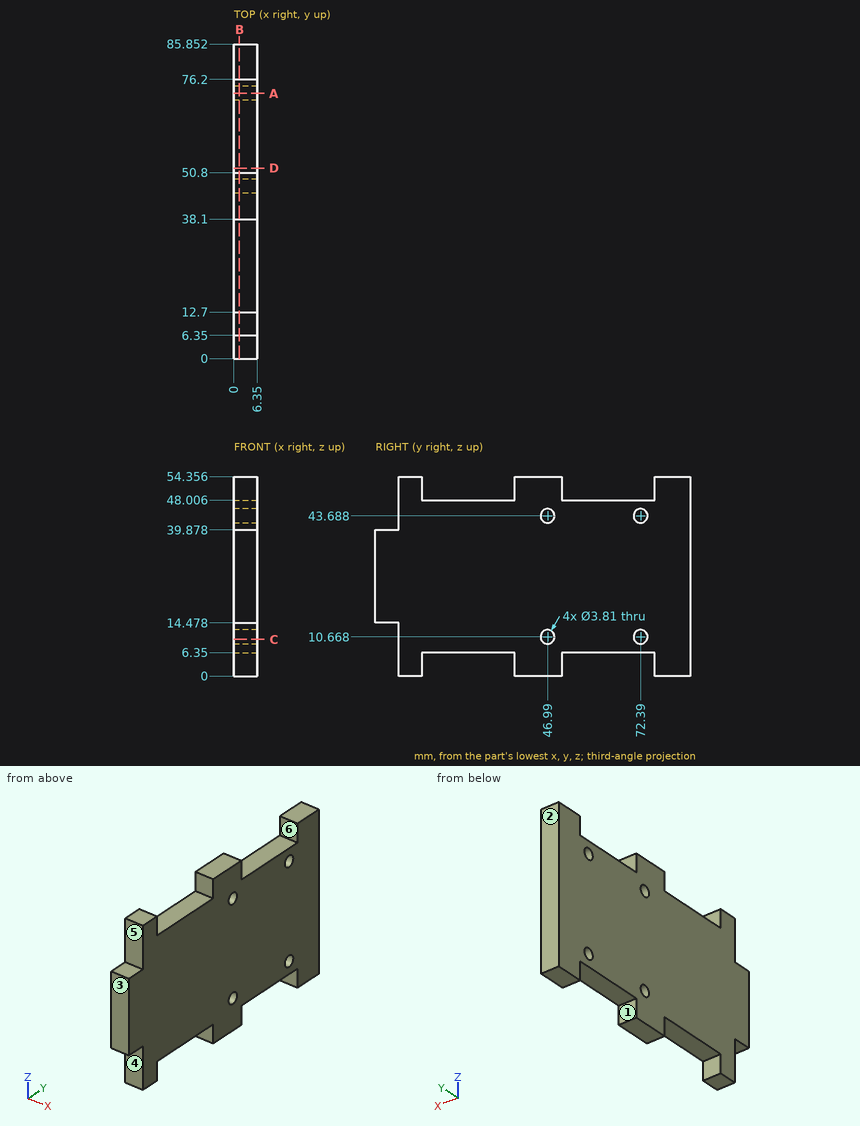
Answer from the drawing. Dimensions are ordinates in mm from the lowest x, y and z of the part. A direction names the side the tool comes from. Round coordinates to 2 decimals unless told otherwise and drop trailing zeros. Write each loop counter-clockwise with the first axis right and the second up, starting at its lowest first coordinate (ties: lowest second). Pieces come first, ordered by that corner, then holes. Notation, with made-up numbers: (32, -12.5) - (78, -12.5) arc R22 ccw to (78, 23.5) - close; hole circle Ø3 at (-12, 74.25). An arc over 180 degrees is marked (long way). Use a Markdown table: item, result.
(1) The part is cut by section A-A (y = 72.39). Write down the section's boundary in (x, z).
Reported:
| item | result |
|---|---|
| outline | (0, 6.35) - (6.35, 6.35) - (6.35, 8.76) - (0, 8.76) - close; (0, 12.57) - (6.35, 12.57) - (6.35, 41.78) - (0, 41.78) - close; (0, 45.59) - (6.35, 45.59) - (6.35, 48.01) - (0, 48.01) - close |
(2) The part is cut by section B-B (x = 1.5). Write down the section's boundary in (y, z) (3 decimals).
Reported:
| item | result |
|---|---|
| outline | (0, 14.478) - (6.35, 14.478) - (6.35, 0) - (12.7, 0) - (12.7, 6.35) - (38.1, 6.35) - (38.1, 0) - (50.8, 0) - (50.8, 6.35) - (76.2, 6.35) - (76.2, 0) - (85.852, 0) - (85.852, 54.356) - (76.2, 54.356) - (76.2, 48.006) - (50.8, 48.006) - (50.8, 54.356) - (38.1, 54.356) - (38.1, 48.006) - (12.7, 48.006) - (12.7, 54.356) - (6.35, 54.356) - (6.35, 39.878) - (0, 39.878) - close; hole circle Ø3.81 at (46.99, 10.668); hole circle Ø3.81 at (46.99, 43.688); hole circle Ø3.81 at (72.39, 10.668); hole circle Ø3.81 at (72.39, 43.688) |
(3) Straight lines are drawn through the part: line 1 along Z through (x, y) = (4.5, 72.39); line 2 along Y through (x, z) = (3.75, 49.5); line 3 along Z through (x, y) = (1.25, 53.5). For each, find the intervals that lie inside material, in ascending order. Write a range as [from, to].
Reported:
| item | result |
|---|---|
| line 1 | [6.35, 8.76], [12.57, 41.78], [45.59, 48.01] |
| line 2 | [6.35, 12.7], [38.1, 50.8], [76.2, 85.85] |
| line 3 | [6.35, 48.01] |
(4) The mould has two halves that part along Y. Classify the marked faces 1, 2 and 3: released by +Y, released by -Y, zero draft, split by the parting line, or undercut.
Reported:
| item | result |
|---|---|
| face 1 | undercut |
| face 2 | released by +Y |
| face 3 | released by -Y |
(5) Each of these flat-tipped pins is pushed along its axis until it touches: pin 1 Ø1.9 at (x, z) = (4.5, 8) entering from -Y; pin 2 Ø1 at (x, z) = (4.5, 31.5) entering from -Y; pin 3 Ø3 at (x, y) = (4.5, 59.5) entering from +Z; pin 4 Ø3 at (x, y) = (3, 19.5) entering from -Z. Where does it stop, or does it pass through?
Reported:
| item | result |
|---|---|
| pin 1 | y = 6.35 |
| pin 2 | y = 0 |
| pin 3 | z = 48.01 |
| pin 4 | z = 6.35 |
(6) The part is cut by section D-D (y = 52). Write down the section's boundary in (x, z), then the cut area to 3 significant figures.
Reported:
| item | result |
|---|---|
| outline | (0, 6.35) - (6.35, 6.35) - (6.35, 48.01) - (0, 48.01) - close |
| area | 265 mm2 |
(7) The part is cut by section C-C (z = 10). Write down the section's boundary in (x, y), then the cut area to 3 significant figures.
Reported:
| item | result |
|---|---|
| outline | (0, 6.35) - (6.35, 6.35) - (6.35, 45.21) - (0, 45.21) - close; (0, 48.77) - (6.35, 48.77) - (6.35, 70.61) - (0, 70.61) - close; (0, 74.17) - (6.35, 74.17) - (6.35, 85.85) - (0, 85.85) - close |
| area | 460 mm2 |
(8) Which of the six approach directions +Z, -Z, +X, -X, +Y, -Y give full straight-line access (tool end or side, diameter ignored) to the marked faces 4, 5 and 6?
Reported:
| item | result |
|---|---|
| face 4 | -Z, +X, -X, -Y |
| face 5 | +Z, +X, -X, -Y |
| face 6 | +Z, +X, -X |
